Here's how the part is built. I have some questions about the finished solid (model axes, mm). Face numbers are marked on the shaded views. A direction names the side the tool comes from. Round coordinates to 2 decimals unless told otherwise and drop trailing zeros. Order: outer loops, then holes, each group sorted by start corner. A loop starts at its lowest first (then second) coordinate and runs counter-clockwise, first axis right, second up. Notation, with made-up numbers: (-20.75, 8) -> (2.25, 8) arc R16 cw to (2.25, 22) -> close; hole circle Ø4 at (-15, 17.5). An arc over 180 degrees is marked (long way). Use a Markdown table: item, result. Add a question column.
(1) I want a section at C-C, the plane y = -37. Please give me the cut outline in (x, z).
(2) I want a section at A-A, the plane x = 115. Please give me the cut outline in (y, z).
(3) If I drill on probe 1 along Y at (x, z) = (23, 9); probe 2 along Z at (x, y) = (32, 4); probe 3 along X at (y, z) = (-18, 32.5), over which ranges is the centre line in solid material (lowest first)?
(4) I want a section at B-B, the plane z = 2. Please give me the cut outline in (x, y).
(5) I'm going to push flat-ended pins straight in: P1, Ø2, axis at y = -79, z = 10, coming from the +X side; P2, Ø10, axis at x = 19.5, z = 5.5, coming from the -Y side; P3, Ø1.5, axis at x = 93.5, z = 13.5, coming from the +Y side; P4, Ø2, axis at y = -91, z = 10, coming from the +X side. Where does each tip first touch, or does it pass through?
(6) I want a section at D-D, the plane x = 64.5. Please give me the cut outline in (y, z), then the cut area to 3 significant figures.
(7) On a 3-axis mill with a long thin cutter (end or side, diameter ignored), from which of +Z, -Z, +X, -X, +Y, -Y can I reach the whole of each face in a straight line? I mean the marked faces 1, 2, 3, 4 and 5. Say none if no direction works.
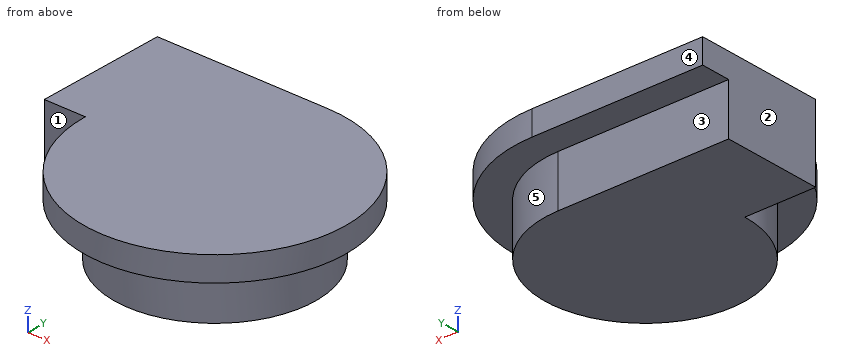
from build123d import *

# Parameters (mm, degrees)
F1_DEPTH = 76.2


with BuildPart() as f1:
    # F0 (on Right) → F1 (new body)
    with BuildSketch(Plane.YZ):
        Polygon((-44.5846021175, 0), (0, 0), (0, 22.8392984718), (13.3088370785, 22.8392984718), (13.3088370785, 33.7528288364), (-44.5846021175, 33.7528288364), align=None)
    extrude(amount=F1_DEPTH)

    # F1_face (on face) → F2 (revolve)
    with BuildSketch(Plane(origin=(76.2, -19.7443345701, 17.881602017), x_dir=(0, 1, 0), z_dir=(1, 0, 0))):
        Polygon((-24.8402675474, -17.881602017), (19.7443345701, -17.881602017), (19.7443345701, 4.9576964548), (33.0531716486, 4.9576964548), (33.0531716486, 15.8712268194), (-24.8402675474, 15.8712268194), align=None)
    revolve(axis=Axis((76.2, -44.5846021175, 16.8764144182), (0, 0, 1)))


solid = f1.part
Taken from the geometry:
| question | item | result |
|---|---|---|
| 1 | outline | (0, 0) -> (120.13, 0) -> (120.13, 22.84) -> (133.59, 22.84) -> (133.59, 33.75) -> (0, 33.75) -> close |
| 2 | outline | (-87.55, 22.84) -> (-66.55, 22.84) -> (-66.55, 0) -> (-22.62, 0) -> (-22.62, 22.84) -> (-1.62, 22.84) -> (-1.62, 33.75) -> (-87.55, 33.75) -> close |
| 3 | probe 1 | y = -44.58 to 0 |
| 3 | probe 2 | z = 22.84 to 33.75 |
| 3 | probe 3 | x = 0 to 127.63 |
| 4 | outline | (0, -44.58) -> (31.62, -44.58) arc R44.58 ccw (long way) to (76.2, 0) -> (0, 0) -> close |
| 5 | P1 | stops at x = 105.72 |
| 5 | P2 | stops at y = -44.58 |
| 5 | P3 | stops at y = -3.19 |
| 5 | P4 | passes through |
| 6 | outline | (-101.28, 22.84) -> (-87.61, 22.84) -> (-87.61, 0) -> (0, 0) -> (0, 22.84) -> (13.31, 22.84) -> (13.31, 33.75) -> (-101.28, 33.75) -> close |
| 6 | area | 3,250 mm2 |
| 7 | face 1 | -Z, -X, -Y |
| 7 | face 2 | +Z, -Z, -X, +Y, -Y |
| 7 | face 3 | -Z, +X, -X, +Y |
| 7 | face 4 | +Z, -Z, +X, -X, +Y |
| 7 | face 5 | -Z |
